```python
from build123d import *

# Parameters (mm, degrees)
SKETCH_2_W               = 12.1
SKETCH_2_H               = 8
EXTRUDE_1_DEPTH          = 12.4
CUT_EXTRUDE_1_DEPTH      = 12.1
CUT_EXTRUDE_2_DEPTH      = 22
CUT_EXTRUDE_2_DEPTH_BACK = 16.1
HOLE_WIZARD_M31_D        = 3.4
HOLE_WIZARD_M31_DEPTH    = 10
HOLE_WIZARD_M31_TIP      = 1.021463052
FILLET_1_R               = 1


with BuildPart() as part:
    # Эскиз2 → Бобышка-Вытянуть1 (new body)
    with BuildSketch(Plane(origin=(0, 0, 0), x_dir=(0, 0, -1), z_dir=(1, 0, 0))):
        Polygon((-19.1, 10), (-19.1, 7), (0, 7), (0, 10), (15.1, 10), (15.1, -20), (12.1, -20), (12.1, 0), (0, 0), (0, -20), (-3, -20), (-3, 0), (-21, 0), (-21, 10), align=None)
        with Locations((6.05, -4)):
            Rectangle(SKETCH_2_W, SKETCH_2_H)
    extrude(amount=EXTRUDE_1_DEPTH)

    # Эскиз3 → Вырез-Вытянуть1 (cut)
    with BuildSketch(Plane.XY):
        with BuildLine():
            Line((0, 0), (-4.310236897, 0))
            Line((-4.310236897, 0), (-4.310236897, -10.158248203))
            Line((-4.310236897, -10.158248203), (16.784307367, -10.158248203))
            Line((16.784307367, -10.158248203), (16.784307367, 0))
            Line((16.784307367, 0), (12.4, 0))
            ThreePointArc((12.4, 0), (6.2, -6.2), (0, 0))
        make_face()
    extrude(amount=-CUT_EXTRUDE_1_DEPTH, mode=Mode.SUBTRACT)

    # Эскиз4 → Вырез-Вытянуть2 (cut, two sides)
    with BuildSketch(Plane.XY) as cut_extrude_2_sk:
        with BuildLine():
            Line((0, -13.8), (-4.529189241, -13.8))
            Line((-4.529189241, -13.8), (-4.529189241, -23.032738442))
            Line((-4.529189241, -23.032738442), (17.457291493, -23.032738442))
            Line((17.457291493, -23.032738442), (17.457291493, -13.8))
            Line((17.457291493, -13.8), (12.4, -13.8))
            ThreePointArc((12.4, -13.8), (6.2, -20), (0, -13.8))
        make_face()
    extrude(amount=CUT_EXTRUDE_2_DEPTH, mode=Mode.SUBTRACT)
    extrude(cut_extrude_2_sk.sketch, amount=-CUT_EXTRUDE_2_DEPTH_BACK, mode=Mode.SUBTRACT)

    # Отверстие с зазором M31
    with Locations(Plane(origin=(0, 7, 0), x_dir=(1, 0, 0), z_dir=(0, 1, 0))):
        with Locations((6.25, -10.05)):
            Hole(HOLE_WIZARD_M31_D / 2, depth=HOLE_WIZARD_M31_DEPTH)
            with Locations((0, 0, -(HOLE_WIZARD_M31_DEPTH + HOLE_WIZARD_M31_TIP / 2))):  # 118° drill point
                Cone(0, HOLE_WIZARD_M31_D / 2, HOLE_WIZARD_M31_TIP, mode=Mode.SUBTRACT)

    # Скругление1
    fillet_1_edges = [part.edges().sort_by_distance(p)[0] for p in [
        (6.2, 0, 21),
        (6.2, 10, 21),
    ]]
    fillet(fillet_1_edges, radius=FILLET_1_R)

    # Эскиз9 → Повернуть1 (revolve)
    with BuildSketch(Plane(origin=(6.2, 0, 0), x_dir=(0, 0, -1), z_dir=(1, 0, 0))):
        with BuildLine():
            Line((12.1, -20), (12.1, -18))
            Line((12.1, -18), (11.3, -18))
            ThreePointArc((11.3, -18), (11.507417596, -19.077032961), (12.1, -20))
        make_face()
    revolve(axis=Axis((6.2, -18, -11.3), (0, 0, -1)))


solid = part.part
```
Part model, mm, in its own coordinate system. A direction names the side the tool comes from. Round coordinates to 2 decimals unless told otherwise and drop trailing zeros. Order: outer loops, then holes, each group sorted by start corner. A loop starts at its lowest first (then second) coordinate and runs counter-clockwise, first axis right, second up. Notation, with made-up numbers: M 30,-24 L 49,-24 A14 ccw 49,-7 Z; hole C -8.5,-30 d4. An arc over 180 degrees is marked long. Put each result on its own line as item: value. Start each with the question number.
1. Drill centre lines: probe 1 along Z at (x, y) = (6.25, 2.25); probe 2 along Z at (x, y) = (11, 7.75); probe 3 along X at (y, z) = (2, 10.05). Where is each one in solid material? Low to high. Write a range as [from, to].
2. Two-plate mould, pull along X, no slides. Class faces 1 (the face through (6.471, 3.451, 8.364)), 2 (the face through (12.4, 1, -1)), 3 (the face through (6, 9, 19.1)), 4 (the face through (6.3, -20, 1.5)): +X half, -X half, draft (parallel to the pull), parting line (faces both ways), or undercut.
3. Drop flat-ended pins along their axis: pin 1 (6 mm diameter, centred on x = 7.5, y = -13.5, fed in from +Z); pin 2 (5 mm diameter, centred on x = 6.5, z = 9.5, fed in from +Y); pin 3 (6 mm diameter, centred on x = 9, z = 9.5, fed in from -Y). Give the stop position or say it passes through.
4. Slice it at D-D on y = -5. List the corners of the cut face in (x, z).
5. Slice it at B-B on y = -8.75. List the corners of the cut face in (x, z), then the cut area to 3 significant figures.
6. Slice it at A-A on z = 10.05. List the corners of the cut face in (x, y).
7. Tool access for faces 5 (the face through (6, -12, -12.1)), 6 (the face through (6, -10, 3)), 7 (the face through (6, 8, 0)): list every direction of +Z, -Z, +X, -X, +Y, -Y with a clear straight run to the whole face (end or side of a thin tool).
8. Slice it at C-C on x = 10.5. List the corners of the cut face in (y, z).
Findings:
1. probe 1: [-15.1, 8.35], [11.75, 21]
1. probe 2: [-15.1, 0], [19.1, 21]
1. probe 3: [0, 4.55], [7.95, 12.4]
2. face 1: undercut
2. face 2: +X half
2. face 3: draft
2. face 4: parting line
3. pin 1: z = 3
3. pin 2: y = 7
3. pin 3: y = 0
4. outline: M 0,-15.1 L 12.4,-15.1 L 12.4,-12.1 L 9.87,-12.1 L 9.87,0 L 12.4,0 L 12.4,3 L 0,3 L 0,0 L 2.53,0 L 2.53,-12.1 L 0,-12.1 Z
5. outline: M 0,-15.1 L 12.4,-15.1 L 12.4,-12.1 L 0,-12.1 Z; M 0,0 L 12.4,0 L 12.4,3 L 0,3 Z
5. area: 74.4 mm2
6. outline: M 0,0 L 4.55,0 L 4.55,7 L 0,7 Z; M 7.95,0 L 12.4,0 L 12.4,7 L 7.95,7 Z
7. face 5: none
7. face 6: +Z, +X, -X, -Y
7. face 7: +X, -X, +Y
8. outline: M -18.27,-15.1 L 10,-15.1 L 10,0 L 7,0 L 7,19.1 L 10,19.1 L 10,20 A1 ccw 9,21 L 1,21 A1 ccw 0,20 L 0,3 L -18.27,3 L -18.27,0 L -4.47,0 L -4.47,-12.1 L -18.27,-12.1 Z
